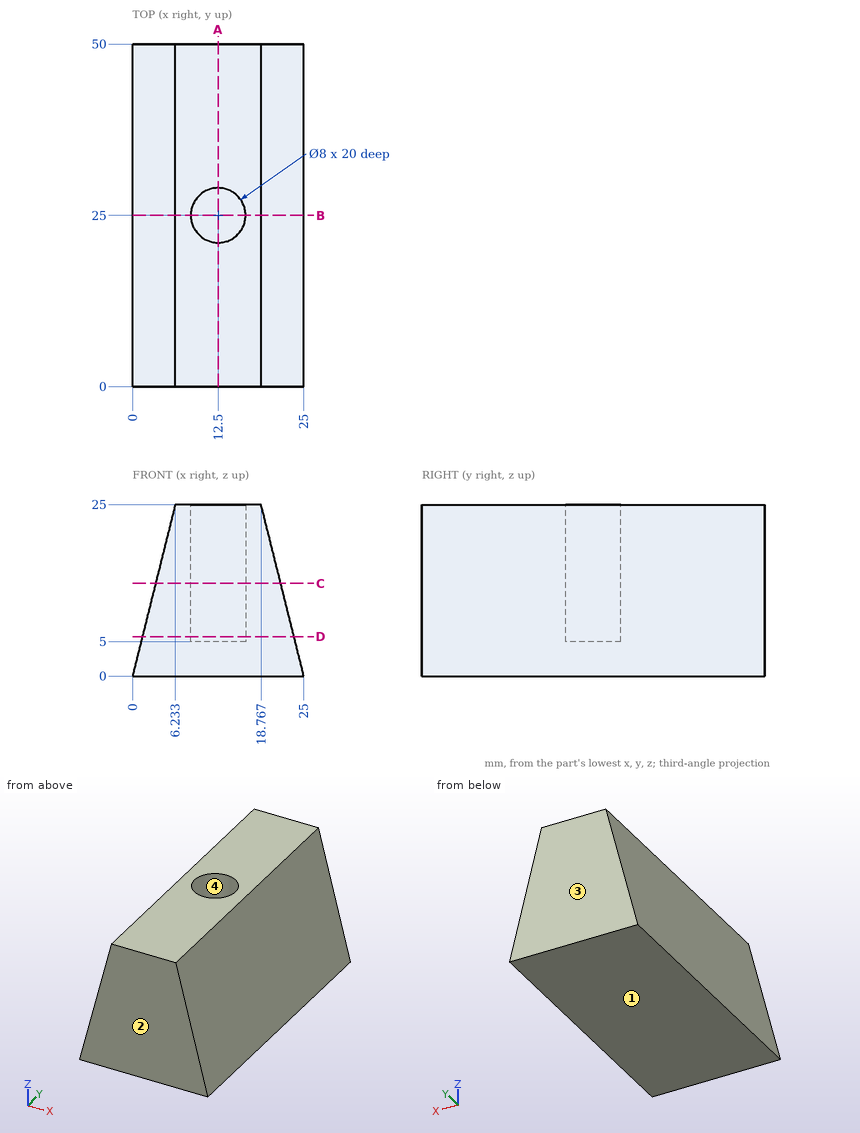
Geometry check sheet. Reference: drawing and pictorial views, mm from the part's lowest x, y, z. Give positions to 0.01 mm unless a question says otherwise; leave off trailing zeros. Write each loop counter-clockwise with the first axis right and the second up, starting at its lowest first coordinate (ties: lowest second). Pieces come first, ordered by that corner, then holes. Notation, with made-up numbers: (-29.75, 30.5) -> (13.25, 30.5) arc R17 ccw to (13.25, 36.5) -> close; hole circle Ø6 at (50.5, 46.5). An arc over 180 degrees is marked (long way). One line per question, with ' | ' between items.
Item 1: Sectioned sample at A-A, the plane x = 12.5. Record the boundary of the cut face in (y, z), plus the area to 3 significant figures.
Determined:
outline: (0, 0) -> (50, 0) -> (50, 25) -> (29, 25) -> (29, 5) -> (21, 5) -> (21, 25) -> (0, 25) -> close | area: 1,090 mm^2
Item 2: Depth check by flat-ended pin: pin 1 (2 mm diameter, centred on y = 29.5, z = 3, fed in from -X); pin 2 (6.5 mm diameter, centred on x = 14, y = 24.5, fed in from +Z). Enter the tip coordinate at first touch or a pass-through.
Determined:
pin 1: x = 0.5 | pin 2: z = 25
Item 3: Sectioned sample at D-D, the plane z = 5.75. Record the boundary of the cut face in (x, y).
Determined:
outline: (1.43, 0) -> (23.57, 0) -> (23.57, 50) -> (1.43, 50) -> close; hole circle Ø8 at (12.5, 25)
Item 4: Scan lines: line 1 along Y through (x, z) = (12.5, 17.25); line 2 along X through (y, z) = (28, 18.5) (1 decimal); line 3 along X through (y, z) = (24.5, 10). Record each from-to range of solid material in increasing order.
Determined:
line 1: 0 to 21, 29 to 50 | line 2: 4.6 to 9.9, 15.1 to 20.4 | line 3: 2.49 to 8.53, 16.47 to 22.51
Item 5: Sectioned sample at B-B, the plane y = 25. Record the boundary of the cut face in (x, z).
Determined:
outline: (0, 0) -> (25, 0) -> (18.77, 25) -> (16.5, 25) -> (16.5, 5) -> (8.5, 5) -> (8.5, 25) -> (6.23, 25) -> close
Item 6: Sectioned sample at C-C, the plane z = 13.5. Record the boundary of the cut face in (x, y), plus the area to 3 significant figures.
Determined:
outline: (3.37, 0) -> (21.63, 0) -> (21.63, 50) -> (3.37, 50) -> close; hole circle Ø8 at (12.5, 25) | area: 863 mm^2
Item 7: Draft check along Y on the marked faces 1, 2, 3 and 4. Enter one of: released by +Y, released by -Y, zero draft, split by the parting line, or undercut.
Determined:
face 1: zero draft | face 2: released by -Y | face 3: released by +Y | face 4: undercut
